```python
from build123d import *

# Parameters (mm, degrees)
SKETCH1_W                     = 18.923
SKETCH1_H                     = 44.323
SKETCH1_R                     = 1.5875
BOSS_EXTRUDE1_DEPTH           = 15.875
FILLET1_R                     = 0.4064
CBORE_FOR_M3_SHCS1_AT_2_COUNT = 2
CBORE_FOR_M3_SHCS1_AT_2_PITCH = 25.4


with BuildPart() as part:
    # Sketch1 → Boss-Extrude1 (new body)
    with BuildSketch(Plane.XY):
        with Locations((9.4615, 22.1615)):
            Rectangle(SKETCH1_W, SKETCH1_H)
        with Locations((9.4615, 9.4615)):
            Circle(SKETCH1_R, mode=Mode.SUBTRACT)
        with Locations((9.4615, 34.8615)):
            Circle(SKETCH1_R, mode=Mode.SUBTRACT)
    extrude(amount=BOSS_EXTRUDE1_DEPTH)

    # Fillet1
    fillet1_edges = [part.edges().sort_by_distance(p)[0] for p in [
        (0, 0, 7.9375),
        (0, 44.323, 7.9375),
        (18.923, 44.323, 7.9375),
        (18.923, 0, 7.9375),
        (7.874, 34.8615, 15.875),
        (9.4615, 0, 15.875),
        (18.923, 22.1615, 15.875),
        (9.4615, 44.323, 15.875),
        (0, 22.1615, 15.875),
        (7.874, 9.4615, 15.875),
    ]]
    fillet(fillet1_edges, radius=FILLET1_R)

    # Sketch2 → CBORE for M3 SHCS1 (revolve, cut)
    with BuildSketch(Plane(origin=(9.4615, 9.4615, 15.875), x_dir=(0, -1, 0), z_dir=(1, 0, 0))):
        Polygon((0, 0), (0, 15.875), (1.6, 15.875), (1.6, 4.5875), (3.25, 4.5875), (3.25, 0.025), (3.275, 0), align=None)
    cbore_for_m3_shcs1 = revolve(axis=Axis((9.4615, 9.4615, 22.225), (0, 0, -1)), mode=Mode.SUBTRACT)

    # CBORE for M3 SHCS1 at 2: CBORE for M3 SHCS1 ×2
    with Locations(*[(0, i * CBORE_FOR_M3_SHCS1_AT_2_PITCH, 0) for i in range(1, CBORE_FOR_M3_SHCS1_AT_2_COUNT)]):
        add(cbore_for_m3_shcs1, mode=Mode.SUBTRACT)


solid = part.part
```
Input: part model. Units: mm. Frame: model coordinates. A direction names the side the tool comes from. Round coordinates to 2 decimals unless told otherwise and drop trailing zeros. Loops run counter-clockwise (first coordinate to the right, second up) from the corner with the lowest first, then second, coordinate; pieces in that order, holes last. Notation, with made-up numbers: (39, 56.25) - (66, 56.25) arc R18 cw to (66, 76.25) - close; hole circle Ø9 at (38.5, -8.75). An arc over 180 degrees is marked (long way). One line per item, written item: value. Start each with the question number.
(1) Access query for faces 4 (the flat face through (9, 22, 0)), 5 (the cylindrical face through (8.49, 6.36, 13.6)). Directions: +Z, -Z, +X, -X, +Y, -Y. A direction counts if a zero-diameter tool reaches every point of the face in a straight line with its end or side. Return the directions, or none.
(2) Draft query along Y for faces 1 (the flat face through (9, 0, 8)), 2 (the flat face through (11, 11, 11.288)), 3 (the flat face through (18.923, 22, 8)). Return one class per face: +Y half, -Y half, draft (parallel to the pull), parting line (faces both ways), or undercut.
(3) Section C-C, the plane z = 14.75. Return loops of the section in (x, y), plus the area to 3 significant figures.
(4) Ray query, line 1 (Y direction, x = 10.25, z = 10.5); line 2 (Y direction, x = 8.75, z = 4.5); line 3 (Z direction, x = 11.5, y = 10). Return the intervals inside material, ascending. Write a range as [from, to].
(5) Contact query for flat-ended pins moving along their axis: P1, Ø1, axis at x = 8.5, y = 8.5, coming from the +Z side; P2, Ø7.5, axis at x = 9.46, y = 9.46, coming from the -Z side. Output: stop coordinate, or through.
(6) Section B-B, the plane x = 10. Count the separate pieces of the cut face and the enclosed holes in it, plus the area to 3 significant figures.
(7) Section A-A, the plane z = 3.75. Return loops of the section in (x, y).
Results below:
1. face 4: -Z, +X, -X, +Y, -Y
1. face 5: +Z
2. face 1: -Y half
2. face 2: undercut
2. face 3: draft
3. outline: (0, 0.41) arc R0.41 ccw to (0.41, 0) - (18.52, 0) arc R0.41 ccw to (18.92, 0.41) - (18.92, 43.92) arc R0.41 ccw to (18.52, 44.32) - (0.41, 44.32) arc R0.41 ccw to (0, 43.92) - close; hole circle Ø6.5 at (9.46, 9.46); hole circle Ø6.5 at (9.46, 34.86)
3. area: 772 mm^2
4. line 1: [0, 8.07], [10.85, 33.47], [36.25, 44.32]
4. line 2: [0, 8.03], [10.89, 33.43], [36.29, 44.32]
4. line 3: [0, 11.29]
5. P1: z = 11.29
5. P2: z = 0
6. separate pieces: 3
6. enclosed holes: 0
6. area: 577 mm^2
7. outline: (0, 0.41) arc R0.41 ccw to (0.41, 0) - (18.52, 0) arc R0.41 ccw to (18.92, 0.41) - (18.92, 43.92) arc R0.41 ccw to (18.52, 44.32) - (0.41, 44.32) arc R0.41 ccw to (0, 43.92) - close; hole circle Ø3.2 at (9.46, 9.46); hole circle Ø3.2 at (9.46, 34.86)
